```python
from build123d import *

# Parameters (mm, degrees)
F1_DEPTH  = 17
F2_W      = 10.8
F2_H      = 15.2113255547
F3_DEPTH  = 3
F4_R      = 1.5
F5_DEPTH  = 20
F8_R      = 2
F9_DEPTH  = 43.2998466183
F11_R     = 2
F12_DEPTH = 43.2998466183
F15_DEPTH = 25
F17_DEPTH = 25
F13_W     = 8
F13_H     = 17
F18_DEPTH = 25


with BuildPart() as f1:
    # F0 (on Front) → F1 (new body, symmetric)
    with BuildSketch(Plane.XZ):
        with BuildLine():
            ThreePointArc((6.7623163428, 20.1020585682), (13.4323577243, 16.4132095267), (18.3675327889, 10.6045))
            Line((18.3675327889, 10.6045), (20.0248161228, 11.5613329789))
            ThreePointArc((20.0248161228, 11.5613329789), (20.9771944934, 12.8595419977), (20.6642504907, 14.4389207581))
            ThreePointArc((20.6642504907, 14.4389207581), (15.7837350444, 19.6562302858), (9.6355470616, 23.2948473664))
            ThreePointArc((9.6355470616, 23.2948473664), (8.7373355906, 24.0314330814), (8.4, 25.1429847274))
            Line((8.4, 25.1429847274), (8.4, 38.209))
            ThreePointArc((8.4, 38.209), (7.8142135624, 39.6232135624), (6.4, 40.209))
            Line((6.4, 40.209), (-6.4, 40.209))
            ThreePointArc((-6.4, 40.209), (-7.8142135624, 39.6232135624), (-8.4, 38.209))
            Line((-8.4, 38.209), (-8.4, 25.1429847274))
            ThreePointArc((-8.4, 25.1429847274), (-8.7373355906, 24.0314330814), (-9.6355470616, 23.2948473664))
            ThreePointArc((-9.6355470616, 23.2948473664), (-15.7837350444, 19.6562302858), (-20.6642504907, 14.4389207581))
            ThreePointArc((-20.6642504907, 14.4389207581), (-20.9771944934, 12.8595419977), (-20.0248161228, 11.5613329789))
            Line((-20.0248161228, 11.5613329789), (-18.3675327889, 10.6045))
            ThreePointArc((-18.3675327889, 10.6045), (-13.4323577243, 16.4132095267), (-6.7623163428, 20.1020585682))
            ThreePointArc((-6.7623163428, 20.1020585682), (-5.7759052807, 20.830491365), (-5.4, 21.9976744453))
            Line((-5.4, 21.9976744453), (-5.4, 37.209))
            Line((-5.4, 37.209), (5.4, 37.209))
            Line((5.4, 37.209), (5.4, 21.9976744453))
            ThreePointArc((5.4, 21.9976744453), (5.7759052807, 20.830491365), (6.7623163428, 20.1020585682))
        make_face()
    extrude(amount=F1_DEPTH, both=True)

    # F2 (on face) → F3 (join)
    with BuildSketch(Plane.XZ.offset(17)):
        with Locations((0, 29.6033372226)):
            Rectangle(F2_W, F2_H)
    extrude(amount=-F3_DEPTH)

    # F4 (on face) → F5 (cut, symmetric)
    with BuildSketch(Plane(origin=(5.4, 0, 0), x_dir=(0, -1, 0), z_dir=(-1, 0, 0))):
        with Locations((-11.2, 23.909)):
            Circle(F4_R)
        with Locations((11, 34.209)):
            Circle(F4_R)
    extrude(amount=F5_DEPTH, both=True, mode=Mode.SUBTRACT)

    # F8 (on line) → F9 (cut, through all)
    with BuildSketch(Plane(origin=(0, 0, 0), x_dir=(0.7071067812, 0, 0.7071067812), z_dir=(0.7071067812, 0, -0.7071067812))):
        Circle(F8_R)
    extrude(amount=-F9_DEPTH, mode=Mode.SUBTRACT)

    # F11 (on line) → F12 (cut, through all)
    with BuildSketch(Plane(origin=(0, 0, 0), x_dir=(0, 1, 0), z_dir=(0.7071067812, 0, 0.7071067812))):
        Circle(F11_R)
    extrude(amount=F12_DEPTH, mode=Mode.SUBTRACT)

    # F14 (on face) → F15 (cut)
    with BuildSketch(Plane.YZ.offset(8.4)):
        with BuildLine():
            Line((12.0528081218, 25.1429847274), (13.6575967311, 25.1429847274))
            ThreePointArc((13.6575967311, 25.1429847274), (11.2, 26.659), (8.7424032689, 25.1429847274))
            Line((8.7424032689, 25.1429847274), (10.3471918782, 25.1429847274))
            ThreePointArc((10.3471918782, 25.1429847274), (11.2, 25.409), (12.0528081218, 25.1429847274))
        make_face()
        with BuildLine():
            ThreePointArc((8.7424032689, 25.1429847274), (10.5659223275, 21.2330991227), (13.95, 23.909))
            ThreePointArc((13.95, 23.909), (13.8759008773, 24.5430776725), (13.6575967311, 25.1429847274))
            Line((13.6575967311, 25.1429847274), (12.0528081218, 25.1429847274))
            ThreePointArc((12.0528081218, 25.1429847274), (11.2, 25.409), (10.3471918782, 25.1429847274))
            Line((10.3471918782, 25.1429847274), (8.7424032689, 25.1429847274))
        make_face()
    extrude(amount=F15_DEPTH, mode=Mode.SUBTRACT)

    # F16 (on face) → F17 (cut)
    with BuildSketch(Plane(origin=(-8.4, 0, 0), x_dir=(0, -1, 0), z_dir=(-1, 0, 0))):
        with BuildLine():
            Line((-12.0528081218, 25.1429847274), (-13.9516602006, 25.1429847274))
            Line((-13.9516602006, 25.1429847274), (-14.6641016151, 23.909))
            Line((-14.6641016151, 23.909), (-12.9320508076, 20.909))
            Line((-12.9320508076, 20.909), (-9.4679491924, 20.909))
            Line((-9.4679491924, 20.909), (-7.7358983849, 23.909))
            Line((-7.7358983849, 23.909), (-8.4483397994, 25.1429847274))
            Line((-8.4483397994, 25.1429847274), (-10.3471918782, 25.1429847274))
            ThreePointArc((-10.3471918782, 25.1429847274), (-11.2, 25.409), (-12.0528081218, 25.1429847274))
        make_face()
    extrude(amount=F17_DEPTH, mode=Mode.SUBTRACT)

    # F13 (on face) → F18 (cut)
    with BuildSketch(Plane.XY.offset(40.209)):
        with Locations((0, 8.5)):
            Rectangle(F13_W, F13_H)
    extrude(amount=-F18_DEPTH, mode=Mode.SUBTRACT)


solid = f1.part
```
Model file for the job. Use its own axes, mm. A direction names the side the tool comes from. Coordinates: 2 decimals unless noted, no trailing zeros. Order: outer loops, then holes, each group sorted by start corner. A loop starts at its lowest first (then second) coordinate and runs counter-clockwise, first axis right, second up. Notation, with made-up numbers: (53.5, 33.25) -> (74.5, 33.25) arc R25 cw to (74.5, 57.25) -> close; hole circle Ø3 at (-32, 81.25). An arc over 180 degrees is marked (long way). Return JSON: item names as keys, results as strings.
Item 1: Mould opens along X. For faces 4 (the face through (5.4, 1, 30)), 5 (the face through (7.83, -0.24, 39.61)), 6 (the face through (-19.21, -0.24, 11.09)), 7 (the face through (6.879, -10.675, 32.745)) say: pulls with the +X half, pulls with the -X half, needs draft (parallel to the pull), parting line crosses it, or undercut.
Model answer:
{"face 4": "undercut", "face 5": "pulls with the +X half", "face 6": "pulls with the -X half", "face 7": "needs draft"}
Item 2: Wall check: line 1 along X through (y, z) = (-3.5, 27.25); line 2 along X through (y, z) = (-7, 13.5); line 3 along Z through (x, y) = (6.65, -11). Give the ranges that are in metal, low to high. Write a range as from..to.
Model answer:
{"line 1": "x = -8.4..-5.4, 5.4..8.4", "line 2": "x = -21.01..-16.36, 16.36..21.01", "line 3": "z = 20.14..32.71, 35.71..40.19"}
Item 3: Pin check, flat tips, straight feed: P1, Ø3.5, axis at y = 11.2, z = 23.909, coming from the -X side; P2, Ø6, axis at y = -6.5, z = 17.5, coming from the -X side; P3, Ø1.5, axis at y = 9, z = 39.5, coming from the +X side. Stop position of each tip, or through.
Model answer:
{"P1": "stops at x = -8.4", "P2": "stops at x = -20.62", "P3": "stops at x = 8.33"}
Item 4: Slice it at A-A (y = -11). Write the cut outline in (x, z).
Model answer:
{"outline": "(-20.66, 14.44) arc R2 ccw to (-20.02, 11.56) -> (-18.37, 10.6) arc R21.21 cw to (-6.76, 20.1) arc R2 ccw to (-5.4, 22) -> (-5.4, 32.71) -> (-8.4, 32.71) -> (-8.4, 25.14) arc R2 cw to (-9.64, 23.29) arc R25.21 ccw to start; (-8.4, 35.71) -> (-5.4, 35.71) -> (-5.4, 37.21) -> (5.4, 37.21) -> (5.4, 35.71) -> (8.4, 35.71) -> (8.4, 38.21) arc R2 ccw to (6.4, 40.21) -> (-6.4, 40.21) arc R2 ccw to (-8.4, 38.21) -> close; (5.4, 22) arc R2 ccw to (6.76, 20.1) arc R21.21 cw to (18.37, 10.6) -> (20.02, 11.56) arc R2 ccw to (20.66, 14.44) arc R25.21 ccw to (9.64, 23.29) arc R2 cw to (8.4, 25.14) -> (8.4, 32.71) -> (5.4, 32.71) -> close"}
Item 5: Slice it at B-B (y = 11.2). Count the separate pieces of the cut face and the enclosed holes in it, then the cut area to 3 significant figures.
Model answer:
{"separate pieces": "4", "enclosed holes": "0", "area": "216 mm²"}
Item 6: Slice it at C-C (z = 26.25). Write the cut outline in (x, y), then the cut area to 3 significant figures.
Model answer:
{"outline": "(-8.4, -17) -> (8.4, -17) -> (8.4, 17) -> (5.4, 17) -> (5.4, -14) -> (-5.4, -14) -> (-5.4, 17) -> (-8.4, 17) -> close", "area": "236 mm²"}
Item 7: 3-axis set-ups, long thin cutter, end or side, ignore diameter. For faces 1 (the face through (-4, 8, 39)), 2 (the face through (-12.161, -0.238, 17.376)), 3 (the face through (-5.4, 1, 29)): which of +Z, -Z, +X, -X, +Y, -Y reach the whole face in a straight line?
Model answer:
{"face 1": "+Z, -Z, +Y", "face 2": "-Z, +Y, -Y", "face 3": "-Z, +Y"}
Item 8: Slice it at D-D (y = -5.5). Write the cut outline in (x, z).
Model answer:
{"outline": "(-20.66, 14.44) arc R2 ccw to (-20.02, 11.56) -> (-18.37, 10.6) arc R21.21 cw to (-6.76, 20.1) arc R2 ccw to (-5.4, 22) -> (-5.4, 37.21) -> (5.4, 37.21) -> (5.4, 22) arc R2 ccw to (6.76, 20.1) arc R21.21 cw to (18.37, 10.6) -> (20.02, 11.56) arc R2 ccw to (20.66, 14.44) arc R25.21 ccw to (9.64, 23.29) arc R2 cw to (8.4, 25.14) -> (8.4, 38.21) arc R2 ccw to (6.4, 40.21) -> (-6.4, 40.21) arc R2 ccw to (-8.4, 38.21) -> (-8.4, 25.14) arc R2 cw to (-9.64, 23.29) arc R25.21 ccw to start"}
